Study the drawing (mm; zero at the part's minimum x, y, z) and answer. Give positions to 0.01 mm unless a question says otherwise; leave off trailing zeros. Order: outer loops, then holes, each group sorted by start corner. A loop starts at its lowest first (then second) coordinate and runs counter-clockwise, first axis right, second up. Notation, with made-up numbers: (11.5, 68.5) - (56.5, 68.5) arc R21 cw to (56.5, 78.5) - close; hole circle Ø3 at (56.25, 29.5). An arc over 180 degrees is marked (long way). Write each question's results on one line, items separated by ' | '. Start each with the question number.
1. Find the intervals of material crossed by L1, parallel to Y at x = 9.5, z = 21; L2, parallel to X at y = 6, z = 19; L3, parallel to Z at x = 22, y = 16.75, in increasing order.
2. Section A-A (x = 19.05) is taken. Give the vertices of the cut face in (y, z).
3. Flat-ended cylindrical pins translate along their axes: pin 1 (4 mm diameter, centred on y = 13.5, z = 13, fed in from -X); pin 2 (1.5 mm diameter, centred on x = 33.5, y = 6.5, fed in from +Z); pin 3 (1 mm diameter, centred on y = 5.5, z = 14, fed in from +X). Find the tip coordinate at first contact, or state that the pin passes through.
4. Determine the mould class of the marked faces 1, 2 and 3 for opening direction Y: released by +Y, released by -Y, zero draft, split by the parting line, or undercut.
5. Section B-B (z = 30.5) is taken. Give the vertices of the cut face in (x, y), and give its area (3 significant figures).
6. Section C-C (x = 33.5) is taken. Give the vertices of the cut face in (y, z).
7. Section D-D (z = 17) is taken. Give the vertices of the cut face in (x, y), and give its area (3 significant figures).
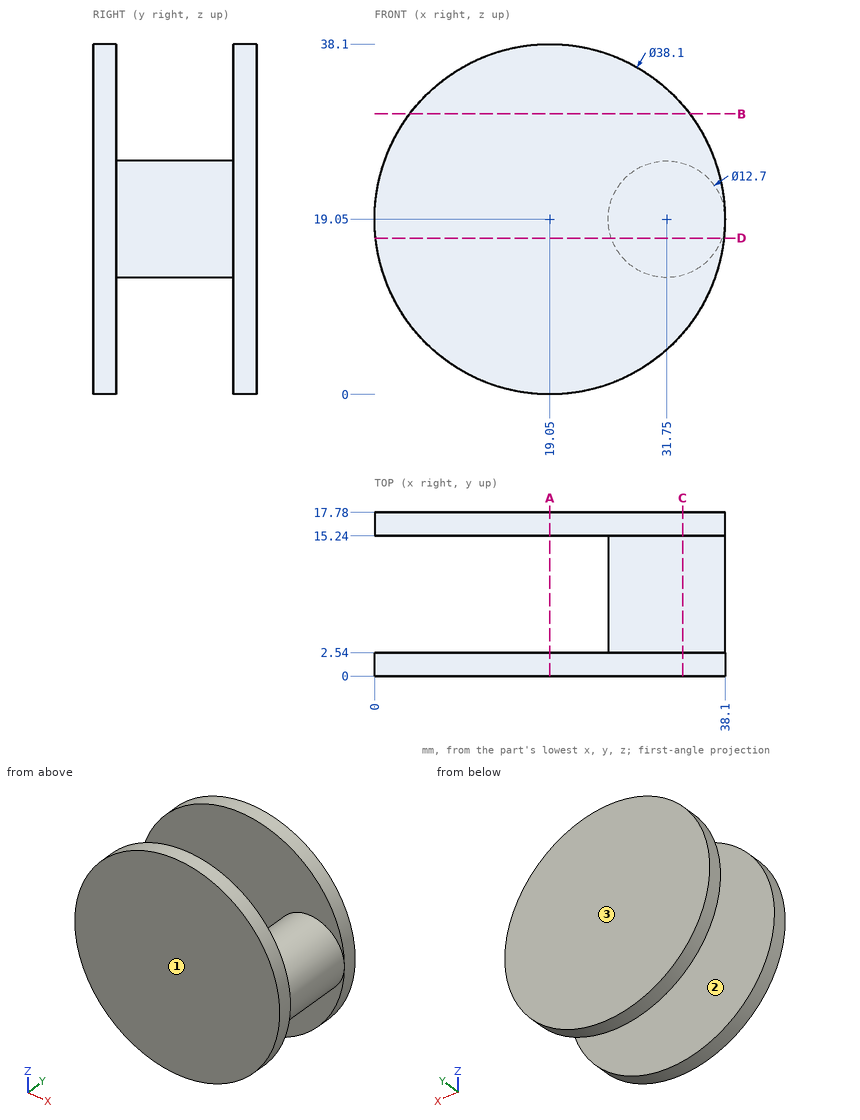
Reported:
1) L1: 0 to 2.54, 15.24 to 17.78 | L2: 25.4 to 38.1 | L3: 0.23 to 37.87
2) outline: (0, 0) - (2.54, 0) - (2.54, 38.1) - (0, 38.1) - close; (15.24, 0) - (17.78, 0) - (17.78, 38.1) - (15.24, 38.1) - close
3) pin 1: x = 0.69 | pin 2: z = 25.32 | pin 3: x = 36.18
4) face 1: released by -Y | face 2: undercut | face 3: released by +Y
5) outline: (3.83, 0) - (34.27, 0) - (34.27, 2.54) - (3.83, 2.54) - close; (3.83, 15.24) - (34.27, 15.24) - (34.27, 17.78) - (3.83, 17.78) - close | area: 155 mm²
6) outline: (0, 6.64) - (2.54, 6.64) - (2.54, 12.95) - (15.24, 12.95) - (15.24, 6.64) - (17.78, 6.64) - (17.78, 31.46) - (15.24, 31.46) - (15.24, 25.15) - (2.54, 25.15) - (2.54, 31.46) - (0, 31.46) - close
7) outline: (0.11, 0) - (37.99, 0) - (37.99, 2.54) - (37.76, 2.54) - (37.76, 15.24) - (37.99, 15.24) - (37.99, 17.78) - (0.11, 17.78) - (0.11, 15.24) - (25.74, 15.24) - (25.74, 2.54) - (0.11, 2.54) - close | area: 345 mm²
